Could you check a few things on this model? Use its own coordinates, in mm. Face numbers are marked on the shaded views. A direction names the side the tool comes from. Coordinates: 2 decimals unless noted, no trailing zeros. Loops run counter-clockwise (first coordinate to the right, second up) from the corner with the lowest first, then second, coordinate; pieces in that order, holes last. Notation, with made-up numbers: M 23.5,42 L 77.5,42 A30 cw 77.5,67 Z; hole C 9,0 d10. An arc over 180 degrees is marked long. Write each question's results on one line, items separated by ' | '.
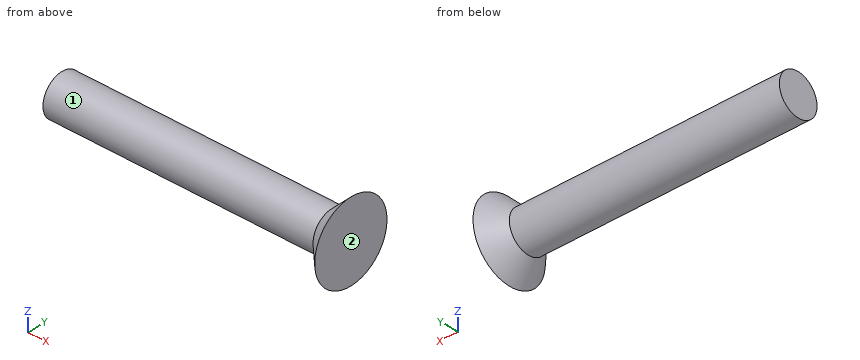
```python
from build123d import *

# Parameters (mm, degrees)
F0_R        = 2.5
F1_DEPTH    = 35
F2_R        = 5
F2_R_2      = 2.5
F3_DEPTH    = 2.8
F4_S5_R     = 2.5
F4_T6_DEPTH = 9


# Not quite as in the source:
# - a fillet or chamfer that OpenCascade refuses, or shapes differently, is made with other operations: its cross-section is extruded or revolved along the edge and cut away or added


with BuildPart() as f1:
    # F0 (on Right) → F1 (new body)
    with BuildSketch(Plane.YZ):
        Circle(F0_R)
    extrude(amount=F1_DEPTH)

    # F2 (on face) → F3 (join)
    with BuildSketch(Plane.YZ.offset(35)):
        Circle(F2_R)
        Circle(F2_R_2, mode=Mode.SUBTRACT)
    extrude(amount=-F3_DEPTH)

    # F4: chamfer of 3 on 1 edges, made by hand


with BuildPart() as f4_tool2:
    # F4_s3 → F4_t4 (revolve)
    with BuildSketch(Plane.XY):
        Polygon((32.2, 2), (35.2, 5), (32.2, 5), align=None)
    revolve(axis=Axis((32.2, 0, 0), (1, 0, 0)))

    # F4_s5 → F4_t6 (cut, symmetric)
    with BuildSketch(Plane.YZ.offset(33.7)):
        Circle(F4_S5_R)
    extrude(amount=F4_T6_DEPTH, both=True, mode=Mode.SUBTRACT)


with BuildPart() as f1_1:
    add(f1.part)

    # F4_t1: cut F4_tool2
    add(f4_tool2.part, mode=Mode.SUBTRACT)


solid = f1_1.part
```
(1) Imagine slicing it at B-B, the plane x = 23.5. List the corners of the cut face in (y, z) for me, and give its area (3 significant figures).
Reported:
outline: C 0,0 d5 | area: 19.6 mm2
(2) Imagine slicing it at A-A, the plane z = 0. List the corners of the cut face in (x, y) for me.
Reported:
outline: M 0,-2.5 L 32.7,-2.5 L 35,-4.8 L 35,4.8 L 32.7,2.5 L 0,2.5 Z
(3) Please list where these lines run through material, in increasing order: probe 1 along Y at (x, z) = (11.5, 0); probe 2 along X at (y, z) = (0.5, 2.5). Write a range as from..to.
Reported:
probe 1: y = -2.5..2.5 | probe 2: x = 32.75..35
(4) Which directions (+Z, -Z, +X, -X, +Y, -Y) give clear straight access to the entire face, cutting with the end or side of a thin tool? Please do the marked faces 1 and 2.
Reported:
face 1: -X | face 2: +Z, -Z, +X, +Y, -Y
(5) Will these pins go through, and if not, where does the flat tip stop? P1, Ø2, axis at x = 22.5, y = 0.5, coming from the -Z side; P2, Ø1.5, axis at x = 30, z = 3, coming from the -Y side; P3, Ø3, axis at x = 17.5, y = -2.5, coming from the -Z side.
Reported:
P1: stops at z = -2.5 | P2: stops at y = -1.09 | P3: stops at z = -2.29
